Here's the drawing with two shaded views (mm, measured from the low corner). I have some questions. A direction names the side the tool comes from. Coordinates: 2 decimals unless noted, no trailing zeros. Loops run counter-clockwise (first coordinate to the right, second up) from the corner with the lowest first, then second, coordinate; pieces in that order, holes last. Notation, with made-up numbers: M 47,70.5 L 98,70.5 A19 cw 98,96.5 Z; hole C 5,-15.5 d9. An arc over 180 degrees is marked long. Use one line per item in the form item = value. Start each with the question number.
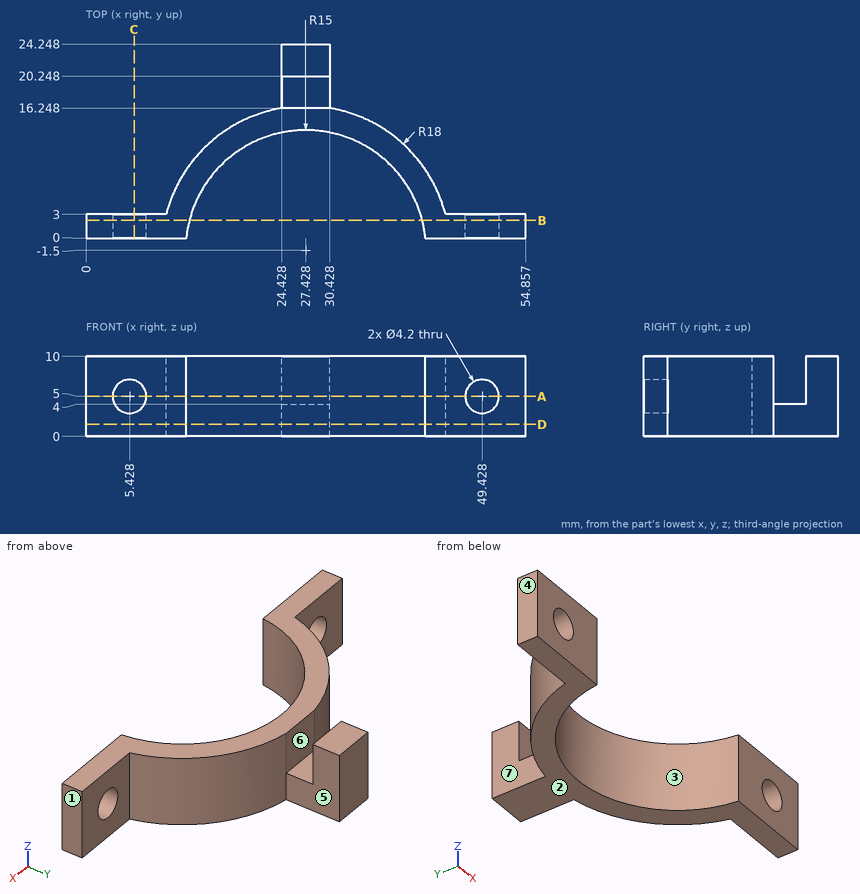
Item 1: I want a section at D-D (z = 1.5). Write out the boundary of the cut face in (x, y), plus the area to 3 significant figures.
Item 2: I want a section at A-A (z = 5). Write out the boundary of the cut face in (x, y).
Item 3: Please list where these lines run through material, in increasing order: line 1 along Y through (x, z) = (28, 9.25); line 2 along Y through (x, z) = (5, 8); line 3 along X through (y, z) = (2.5, 0.75) (1 decimal).
Item 4: I want a section at B-B (y = 2.25). Write out the boundary of the cut face in (x, z) (1 decimal).
Item 5: For the marked faces 5, 6 and 7, which set-ups out of +Z, -Z, +X, -X, +Y, -Y let a thin tool reach every point of the face, with its end or its side?
Item 6: I want a section at C-C (x = 6). Write out the boundary of the cut face in (y, z), plus the area to 3 significant figures.
Item 7: Thinking about a two-plate mould opening in X: for the marked faces 1, 2, 3 and 4, which applies, pulls with the +X half, pulls with the -X half, needs draft (parallel to the pull), parting line crosses it, or undercut?
Item 8: I'm going to push flat-ended pins straight in: P1, Ø1.8, axis at x = 28, z = 6.5, coming from the -Y side; P2, Ø5, axis at x = 51.5, z = 4.5, coming from the +Y side; P3, Ø5, axis at x = 16.5, z = 5, coming from the +Y side (1 decimal); P4, Ø4, axis at x = 5.43, z = 5, coming from the -Y side. Where does each tip first touch, or does it pass through?
Worked answers:
q1.outline = M 0,0 L 12.5,0 A15 cw 42.35,0 L 54.86,0 L 54.86,3 L 44.86,3 A18 ccw 30.43,16.25 L 30.43,24.25 L 24.43,24.25 L 24.43,16.25 A18 ccw 10,3 L 0,3 Z
q1.area = 252 mm²
q2.outline = M 0,0 L 3.33,0 L 3.33,3 L 0,3 Z; M 7.53,0 L 12.5,0 A15 cw 42.35,0 L 47.33,0 L 47.33,3 L 44.86,3 A18 ccw 30.43,16.25 L 24.43,16.25 A18 ccw 10,3 L 7.53,3 Z; M 24.43,20.25 L 30.43,20.25 L 30.43,24.25 L 24.43,24.25 Z; M 51.53,0 L 54.86,0 L 54.86,3 L 51.53,3 Z
q3.line_1 = 13.49 to 16.25, 20.25 to 24.25
q3.line_2 = 0 to 3
q3.line_3 = 0 to 13, 41.9 to 54.9
q4.outline = M 0,0 L 12.9,0 L 12.9,10 L 0,10 Z; M 42,0 L 54.9,0 L 54.9,10 L 42,10 Z; hole C 5.4,5 d4.2; hole C 49.4,5 d4.2
q5.face_5 = +Z, -Z, +X, +Y
q5.face_6 = +Z, +X, -X
q5.face_7 = +Z, -Z, -X, +Y
q6.outline = M 0,0 L 3,0 L 3,2.98 L 0,2.98 Z; M 0,7.02 L 3,7.02 L 3,10 L 0,10 Z
q6.area = 17.9 mm²
q7.face_1 = pulls with the +X half
q7.face_2 = needs draft
q7.face_3 = undercut
q7.face_4 = pulls with the -X half
q8.P1 = 13.43
q8.P2 = 3
q8.P3 = 14.4
q8.P4 = through
